Part model, mm, in its own coordinate system. A direction names the side the tool comes from. Coordinates: 2 decimals unless noted, no trailing zeros. Write each loop counter-clockwise with the first axis right and the second up, starting at its lowest first coordinate (ties: lowest second). Pieces come first, ordered by that corner, then holes. Notation, with made-up numbers: (75, 32) - (123, 32) arc R25 ccw to (123, 65) - close; hole circle Ø8 at (59.25, 68). An arc over 180 degrees is marked (long way). Use a Markdown table: item, result.
```python
from build123d import *

# Parameters (mm, degrees)
SKETCH1_W            = 33
SKETCH1_H            = 41.24
BOSS_EXTRUDE1_DEPTH  = 1.59
M3_CLEARANCE_HOLE1_D = 3.3
SKETCH6_W            = 16
SKETCH6_H            = 12.2
M8P_DEPTH            = 2.4
SKETCH7_W            = 6
SKETCH7_H            = 4.25
I2C_CONNECTORS_DEPTH = 3.14


with BuildPart() as part:
    # Sketch1 → Boss-Extrude1 (new body)
    with BuildSketch(Plane(origin=(0, 0, 0), x_dir=(1, 0, 0), z_dir=(0, 1, 0))):
        Rectangle(SKETCH1_W, SKETCH1_H)
    extrude(amount=BOSS_EXTRUDE1_DEPTH)

    # M3 Clearance Hole1 (through all)
    with Locations(Plane(origin=(0, 1.59, 0), x_dir=(1, 0, 0), z_dir=(0, 1, 0))):
        with Locations((-13.97, 17.78), (13.97, 17.78), (13.97, -17.78), (-13.97, -17.78)):
            Hole(M3_CLEARANCE_HOLE1_D / 2)

    # Sketch6 → M8P (add)
    with BuildSketch(Plane(origin=(0, 1.59, 0), x_dir=(1, 0, 0), z_dir=(0, 1, 0))):
        Rectangle(SKETCH6_W, SKETCH6_H)
    extrude(amount=M8P_DEPTH)

    # Sketch7 → I2C connectors (add)
    with BuildSketch(Plane(origin=(0, 1.59, 0), x_dir=(1, 0, 0), z_dir=(0, 1, 0))):
        with Locations((0, -17.695)):
            Rectangle(SKETCH7_W, SKETCH7_H)
        with Locations((0, 17.695)):
            Rectangle(SKETCH7_W, SKETCH7_H)
    extrude(amount=I2C_CONNECTORS_DEPTH)


solid = part.part
```
Item 1: Two-plate mould, pull along X, no slides. Class faces 4 (the face through (15.62, 0.78, 17.71)), 5 (the face through (0, 4.73, -18)), 6 (the face through (15.186, 0.784, -18.895)), 7 (the face through (-8, 3, 0)): pulls with the +X half, pulls with the -X half, needs draft (parallel to the pull), parting line crosses it, or undercut.
From the geometry:
| item | result |
|---|---|
| face 4 | undercut |
| face 5 | needs draft |
| face 6 | undercut |
| face 7 | pulls with the -X half |
Item 2: Which spindle directions (+Z, -Z, +X, -X, +Y, -Y) get a long thin tool onto all of the face, cutting with end or side? Do faces 1 (the face through (0, 3.99, 0)), 2 (the face through (3, 3, 18)), 3 (the face through (3, 3, -18)). Say none if no direction does.
From the geometry:
| item | result |
|---|---|
| face 1 | +X, -X, +Y |
| face 2 | +Z, +X, +Y |
| face 3 | -Z, +X, +Y |
Item 3: Band-saw the part on C-C, the plane y = 1. Give the cut face in (x, z).
From the geometry:
| item | result |
|---|---|
| outline | (-16.5, -20.62) - (16.5, -20.62) - (16.5, 20.62) - (-16.5, 20.62) - close; hole circle Ø3.3 at (-13.97, -17.78); hole circle Ø3.3 at (-13.97, 17.78); hole circle Ø3.3 at (13.97, -17.78); hole circle Ø3.3 at (13.97, 17.78) |
Item 4: Drop flat-ended pins along their axis: P1, Ø2, axis at x = 8.5, z = -4.5, coming from the +Y side; P2, Ø5.5, axis at x = 13.97, z = -17.78, coming from the +Y side; P3, Ø2.5, axis at x = 1, y = 3, coming from the -Z side; P4, Ø2, axis at y = 4, z = 7.5, coming from the -X side. Give the stop position or say it passes through.
From the geometry:
| item | result |
|---|---|
| P1 | y = 3.99 |
| P2 | y = 1.59 |
| P3 | z = -19.82 |
| P4 | through |
Item 5: Band-saw the part on A-A, the plane z = 17.78. Give the cut face in (x, y), then the cut area to 3 significant figures.
From the geometry:
| item | result |
|---|---|
| outline | (-16.5, 0) - (-15.62, 0) - (-15.62, 1.59) - (-16.5, 1.59) - close; (-12.32, 0) - (12.32, 0) - (12.32, 1.59) - (3, 1.59) - (3, 4.73) - (-3, 4.73) - (-3, 1.59) - (-12.32, 1.59) - close; (15.62, 0) - (16.5, 0) - (16.5, 1.59) - (15.62, 1.59) - close |
| area | 60.8 mm^2 |
Item 6: Drill centre lines: probe 1 along X at (y, z) = (1.1, 17.78); probe 2 along Z at (x, y) = (13.97, 0.5); probe 3 along X at (y, z) = (3.4, 5). Where is each one in solid material? Low to high.
From the geometry:
| item | result |
|---|---|
| probe 1 | -16.5 to -15.62, -12.32 to 12.32, 15.62 to 16.5 |
| probe 2 | -20.62 to -19.43, -16.13 to 16.13, 19.43 to 20.62 |
| probe 3 | -8 to 8 |
Item 7: Band-saw the part on B-B, the plane x = -13.97. Give the cut face in (y, z), then the cut area to 3 significant figures.
From the geometry:
| item | result |
|---|---|
| outline | (0, -20.62) - (1.59, -20.62) - (1.59, -19.43) - (0, -19.43) - close; (0, -16.13) - (1.59, -16.13) - (1.59, 16.13) - (0, 16.13) - close; (0, 19.43) - (1.59, 19.43) - (1.59, 20.62) - (0, 20.62) - close |
| area | 55.1 mm^2 |
Item 8: Band-saw the part on D-D, the plane z = -3. Give the cut face in (x, y), then the cut area to 3 significant figures.
From the geometry:
| item | result |
|---|---|
| outline | (-16.5, 0) - (16.5, 0) - (16.5, 1.59) - (8, 1.59) - (8, 3.99) - (-8, 3.99) - (-8, 1.59) - (-16.5, 1.59) - close |
| area | 90.9 mm^2 |
